from build123d import *
from build123d.topology import SkipClean

# Parameters (mm, degrees)
SKETCH2_W                                            = 92.5
SKETCH2_H                                            = 42
SKETCH2_R                                            = 3.2
BOSS_EXTRUDE1_DEPTH                                  = 6
M3_CLEARANCE_HOLE1_D                                 = 3.6
M3_CLEARANCE_HOLE1_DEPTH                             = 10
M3_CLEARANCE_HOLE1_TIP                               = 1.081549114
BOSS_EXTRUDE2_START                                  = 3
SKETCH7_R                                            = 7.2
SKETCH7_R_2                                          = 3.2
BOSS_EXTRUDE2_DEPTH                                  = 3
CHAMFER1_SIZE                                        = 3
FILLET1_R                                            = 3
CSK_FOR_M3_HEX_SOCKET_COUNTERSUNK_HEAD_S_D           = 3.6
CSK_FOR_M3_HEX_SOCKET_COUNTERSUNK_HEAD_S_CSINK_D     = 6.94
CSK_FOR_M3_HEX_SOCKET_COUNTERSUNK_HEAD_S_CSINK_ANGLE = 90


with BuildPart() as part:
    # Sketch2 → Boss-Extrude1 (new body)
    with BuildSketch(Plane(origin=(0, 0, 0), x_dir=(1, 0, 0), z_dir=(0, 1, 0))):
        with Locations((20.253338886, 13.715343577)):
            Rectangle(SKETCH2_W, SKETCH2_H)
        with Locations(Location((20.253338886, 13.715343577, 0), (0, 0, 270))):
            Circle(SKETCH2_R, mode=Mode.SUBTRACT)
    extrude(amount=BOSS_EXTRUDE1_DEPTH)

    # M3 Clearance Hole1
    with Locations(Plane(origin=(0, 0, 0), x_dir=(-1, 0, 0), z_dir=(0, -1, 0))):
        with Locations((-60.253338886, 27.515343577), (-60.253338886, -2.984656423), (19.746661114, -2.984656423), (19.746661114, 27.515343577)):
            Hole(M3_CLEARANCE_HOLE1_D / 2, depth=M3_CLEARANCE_HOLE1_DEPTH)
            with Locations((0, 0, -(M3_CLEARANCE_HOLE1_DEPTH + M3_CLEARANCE_HOLE1_TIP / 2))):  # 118° drill point
                Cone(0, M3_CLEARANCE_HOLE1_D / 2, M3_CLEARANCE_HOLE1_TIP, mode=Mode.SUBTRACT)

    # Sketch7 → Boss-Extrude2 (add)
    with SkipClean():  # the faces are left unmerged after this step: merging them gives an invalid solid
        with BuildSketch(Plane.XZ.offset(BOSS_EXTRUDE2_START)):
            with Locations(Location((20.253338886, -13.715343577, 0), (0, 0, 90))):
                Circle(SKETCH7_R)
            with Locations(Location((20.253338886, -13.715343577, 0), (0, 0, 270))):
                Circle(SKETCH7_R_2, mode=Mode.SUBTRACT)
        extrude(amount=-BOSS_EXTRUDE2_DEPTH)

    # Chamfer1
    chamfer1_edges = [part.edges().sort_by_distance(p)[0] for p in [
        (20.253338886, 0, -20.915343577),
    ]]
    chamfer(chamfer1_edges, length=CHAMFER1_SIZE - 0.0001)  # a hair under: the kernel refuses the full size

    # Fillet1
    fillet1_edges = [part.edges().sort_by_distance(p)[0] for p in [
        (-25.996661114, 3, -34.715343577),
        (66.503338886, 3, -34.715343577),
        (66.503338886, 3, 7.284656423),
        (-25.996661114, 3, 7.284656423),
    ]]
    fillet(fillet1_edges, radius=FILLET1_R)

    # CSK for M3 Hex Socket Countersunk Head Screw1 (through all)
    with Locations(Plane(origin=(0, 0, 0), x_dir=(-1, 0, 0), z_dir=(0, -1, 0))):
        with Locations((-59.503338886, 13.715343577), (18.996661114, 13.715343577)):
            CounterSinkHole(CSK_FOR_M3_HEX_SOCKET_COUNTERSUNK_HEAD_S_D / 2, CSK_FOR_M3_HEX_SOCKET_COUNTERSUNK_HEAD_S_CSINK_D / 2, counter_sink_angle=CSK_FOR_M3_HEX_SOCKET_COUNTERSUNK_HEAD_S_CSINK_ANGLE)


solid = part.part
Input: part model. Units: mm. Frame: model coordinates. Give positions to 0.01 mm unless a question says otherwise; leave off trailing zeros. Write each loop counter-clockwise with the first axis right and the second up, starting at its lowest first coordinate (ties: lowest second). Pieces come first, ordered by that corner, then holes.
Q1. Material intervals for probe 1 along X at (y, z) = (4.5, 3); probe 2 along X at (y, z) = (3, 4); probe 3 along X at (y, z) = (1.25, -12.5), sorted ascending.
Q2. Section A-A, the plane y = 3.5. Output: boundary loops of the cut face in (x, z).
Q3. Pull-direction query (Z, two-part tool) for faces 1 (the face through (-25.141, 3.042, 6.383)), 2 (the face through (66.503, 3, -13)), 3 (the face through (61.97, 3.04, 2.44)), 4 (the face through (-25.141, 3.042, -33.813)); classes: pulls with the +Z half, pulls with the -Z half, needs draft (parallel to the pull), parting line crosses it, or undercut.
Q4. Section B-B, the plane z = -0.5. Output: boundary loops of the cut face in (x, y), plus the area to 3 significant figures.
Q5. First-contact query: P1, Ø4.5, axis at x = 59.5, z = -13.72, coming from the +Y side; P2, Ø4.5, axis at x = -19.75, z = -27.52, coming from the -Y side; P3, Ø4, axis at x = -19, z = -13.72, coming from the -Y side; P4, Ø5, axis at x = 20.25, z = -13.72, coming from the -Y side. Flat tips, straight axial feed; report the tip coordinate or a pass-through.
Q6. Section C-C, the plane x = -14. Output: boundary loops of the cut face in (y, z).
Filled in:
1. probe 1: x = -26 to -21.55, -17.95 to 58.45, 62.05 to 66.5
1. probe 2: x = -26 to -21.23, -18.26 to 58.77, 61.74 to 66.5
1. probe 3: x = -26 to -20.85, -17.14 to 17.29, 23.21 to 57.65, 61.36 to 66.5
2. outline: (-26, -31.72) arc R3 ccw to (-23, -34.72) - (63.5, -34.72) arc R3 ccw to (66.5, -31.72) - (66.5, 4.28) arc R3 ccw to (63.5, 7.28) - (-23, 7.28) arc R3 ccw to (-26, 4.28) - close; hole circle Ø3.6 at (-19.75, -27.52); hole circle Ø3.6 at (-19.75, 2.98); hole circle Ø3.6 at (-19, -13.72); hole circle Ø6.4 at (20.25, -13.72); hole circle Ø3.6 at (59.5, -13.72); hole circle Ø3.6 at (60.25, -27.52); hole circle Ø3.6 at (60.25, 2.98)
3. face 1: pulls with the +Z half
3. face 2: needs draft
3. face 3: undercut
3. face 4: pulls with the -Z half
4. outline: (-26, 0) - (66.5, 0) - (66.5, 6) - (-26, 6) - close
4. area: 555 mm2
5. P1: stops at y = 6
5. P2: stops at y = 0
5. P3: stops at y = 1.46
5. P4: passes through
6. outline: (0, -34.72) - (6, -34.72) - (6, 7.28) - (0, 7.28) - close
